from build123d import *

# Parameters (mm, degrees)
SKETCH2_R               = 34
BOSS_EXTRUDE1_DEPTH     = 5
CUT_EXTRUDE_THIN1_REACH = 50.343
CUT_EXTRUDE1_REACH      = 50.343
SKETCH7_R               = 1.5
CUT_EXTRUDE2_REACH      = 50.343
SKETCH8_R               = 3.5
SKETCH9_R               = 30
CUT_EXTRUDE3_DEPTH      = 2


with BuildPart() as part:
    # Sketch2 → Boss-Extrude1 (new body)
    with BuildSketch(Plane.XY):
        Circle(SKETCH2_R)
    extrude(amount=BOSS_EXTRUDE1_DEPTH)

    # Sketch3 → Cut-Extrude-Thin1 (cut, up to next)
    with BuildSketch(Plane.XY.offset(5), mode=Mode.PRIVATE) as cut_extrude_thin1_sk1:
        with BuildLine():
            ThreePointArc((0, 25.5), (18, 7.5), (0, -10.5))
            Line((0, -10.5), (0, -17.5))
            ThreePointArc((0, -17.5), (25, 7.5), (0, 32.5))
            Line((0, 32.5), (0, 25.5))
        make_face()
    cut_extrude_thin1_tool1 = extrude(cut_extrude_thin1_sk1.sketch, amount=-CUT_EXTRUDE_THIN1_REACH, mode=Mode.PRIVATE) & part.part
    # Sketch3 → Cut-Extrude-Thin1 (cut, up to next)
    with BuildSketch(Plane.XY.offset(5), mode=Mode.PRIVATE) as cut_extrude_thin1_sk2:
        with BuildLine():
            ThreePointArc((22.083647797, -12.75), (-2.504809472, -19.338457268), (-9.09326674, 5.25))
            Line((-9.09326674, 5.25), (-15.155444566, 8.75))
            ThreePointArc((-15.155444566, 8.75), (-6.004809472, -25.400635095), (28.145825623, -16.25))
            Line((28.145825623, -16.25), (22.083647797, -12.75))
        make_face()
    cut_extrude_thin1_tool2 = extrude(cut_extrude_thin1_sk2.sketch, amount=-CUT_EXTRUDE_THIN1_REACH, mode=Mode.PRIVATE) & part.part
    # Sketch3 → Cut-Extrude-Thin1 (cut, up to next)
    with BuildSketch(Plane.XY.offset(5), mode=Mode.PRIVATE) as cut_extrude_thin1_sk3:
        with BuildLine():
            ThreePointArc((-22.083647797, -12.75), (-15.495190528, 11.838457268), (9.09326674, 5.25))
            Line((9.09326674, 5.25), (15.155444566, 8.75))
            ThreePointArc((15.155444566, 8.75), (-18.995190528, 17.900635095), (-28.145825623, -16.25))
            Line((-28.145825623, -16.25), (-22.083647797, -12.75))
        make_face()
    cut_extrude_thin1_tool3 = extrude(cut_extrude_thin1_sk3.sketch, amount=-CUT_EXTRUDE_THIN1_REACH, mode=Mode.PRIVATE) & part.part
    add(cut_extrude_thin1_tool1.solids().sort_by_distance((0.559017, 29, 5))[0], mode=Mode.SUBTRACT)
    add(cut_extrude_thin1_tool2.solids().sort_by_distance((-2.804081, -19.85681, 5))[0], mode=Mode.SUBTRACT)
    add(cut_extrude_thin1_tool3.solids().sort_by_distance((-15.794462, 12.35681, 5))[0], mode=Mode.SUBTRACT)

    # Sketch7 → Cut-Extrude1 (cut, up to next)
    with BuildSketch(Plane(origin=(0, 0, 0), x_dir=(-1, 0, 0), z_dir=(0, 0, -1)), mode=Mode.PRIVATE) as cut_extrude1_sk1:
        with Locations((7, 0)):
            Circle(SKETCH7_R)
    cut_extrude1_tool1 = extrude(cut_extrude1_sk1.sketch, amount=-CUT_EXTRUDE1_REACH, mode=Mode.PRIVATE) & part.part
    # Sketch7 → Cut-Extrude1 (cut, up to next)
    with BuildSketch(Plane(origin=(0, 0, 0), x_dir=(-1, 0, 0), z_dir=(0, 0, -1)), mode=Mode.PRIVATE) as cut_extrude1_sk2:
        with Locations((0, -7)):
            Circle(SKETCH7_R)
    cut_extrude1_tool2 = extrude(cut_extrude1_sk2.sketch, amount=-CUT_EXTRUDE1_REACH, mode=Mode.PRIVATE) & part.part
    # Sketch7 → Cut-Extrude1 (cut, up to next)
    with BuildSketch(Plane(origin=(0, 0, 0), x_dir=(-1, 0, 0), z_dir=(0, 0, -1)), mode=Mode.PRIVATE) as cut_extrude1_sk3:
        with Locations((-7, 0)):
            Circle(SKETCH7_R)
    cut_extrude1_tool3 = extrude(cut_extrude1_sk3.sketch, amount=-CUT_EXTRUDE1_REACH, mode=Mode.PRIVATE) & part.part
    # Sketch7 → Cut-Extrude1 (cut, up to next)
    with BuildSketch(Plane(origin=(0, 0, 0), x_dir=(-1, 0, 0), z_dir=(0, 0, -1)), mode=Mode.PRIVATE) as cut_extrude1_sk4:
        with Locations((0, 7)):
            Circle(SKETCH7_R)
    cut_extrude1_tool4 = extrude(cut_extrude1_sk4.sketch, amount=-CUT_EXTRUDE1_REACH, mode=Mode.PRIVATE) & part.part
    add(cut_extrude1_tool1.solids().sort_by_distance((-7, 0, 0))[0], mode=Mode.SUBTRACT)
    add(cut_extrude1_tool2.solids().sort_by_distance((0, -7, 0))[0], mode=Mode.SUBTRACT)
    add(cut_extrude1_tool3.solids().sort_by_distance((7, 0, 0))[0], mode=Mode.SUBTRACT)
    add(cut_extrude1_tool4.solids().sort_by_distance((0, 7, 0))[0], mode=Mode.SUBTRACT)

    # Sketch8 → Cut-Extrude2 (cut, up to next)
    with BuildSketch(Plane(origin=(0, 0, 0), x_dir=(-1, 0, 0), z_dir=(0, 0, -1)), mode=Mode.PRIVATE) as cut_extrude2_sk1:
        with Locations((0, 29)):
            Circle(SKETCH8_R)
    cut_extrude2_tool1 = extrude(cut_extrude2_sk1.sketch, amount=-CUT_EXTRUDE2_REACH, mode=Mode.PRIVATE) & part.part
    # Sketch8 → Cut-Extrude2 (cut, up to next)
    with BuildSketch(Plane(origin=(0, 0, 0), x_dir=(-1, 0, 0), z_dir=(0, 0, -1)), mode=Mode.PRIVATE) as cut_extrude2_sk2:
        with Locations((-12.124355653, 7)):
            Circle(SKETCH8_R)
    cut_extrude2_tool2 = extrude(cut_extrude2_sk2.sketch, amount=-CUT_EXTRUDE2_REACH, mode=Mode.PRIVATE) & part.part
    # Sketch8 → Cut-Extrude2 (cut, up to next)
    with BuildSketch(Plane(origin=(0, 0, 0), x_dir=(-1, 0, 0), z_dir=(0, 0, -1)), mode=Mode.PRIVATE) as cut_extrude2_sk3:
        with Locations((12.124355653, 7)):
            Circle(SKETCH8_R)
    cut_extrude2_tool3 = extrude(cut_extrude2_sk3.sketch, amount=-CUT_EXTRUDE2_REACH, mode=Mode.PRIVATE) & part.part
    # Sketch8 → Cut-Extrude2 (cut, up to next)
    with BuildSketch(Plane(origin=(0, 0, 0), x_dir=(-1, 0, 0), z_dir=(0, 0, -1)), mode=Mode.PRIVATE) as cut_extrude2_sk4:
        with Locations((25.11473671, -14.5)):
            Circle(SKETCH8_R)
    cut_extrude2_tool4 = extrude(cut_extrude2_sk4.sketch, amount=-CUT_EXTRUDE2_REACH, mode=Mode.PRIVATE) & part.part
    # Sketch8 → Cut-Extrude2 (cut, up to next)
    with BuildSketch(Plane(origin=(0, 0, 0), x_dir=(-1, 0, 0), z_dir=(0, 0, -1)), mode=Mode.PRIVATE) as cut_extrude2_sk5:
        with Locations((-25.11473671, -14.5)):
            Circle(SKETCH8_R)
    cut_extrude2_tool5 = extrude(cut_extrude2_sk5.sketch, amount=-CUT_EXTRUDE2_REACH, mode=Mode.PRIVATE) & part.part
    # Sketch8 → Cut-Extrude2 (cut, up to next)
    with BuildSketch(Plane(origin=(0, 0, 0), x_dir=(-1, 0, 0), z_dir=(0, 0, -1)), mode=Mode.PRIVATE) as cut_extrude2_sk6:
        with Locations((0, -14)):
            Circle(SKETCH8_R)
    cut_extrude2_tool6 = extrude(cut_extrude2_sk6.sketch, amount=-CUT_EXTRUDE2_REACH, mode=Mode.PRIVATE) & part.part
    add(cut_extrude2_tool1.solids().sort_by_distance((0, 29, 0))[0], mode=Mode.SUBTRACT)
    add(cut_extrude2_tool2.solids().sort_by_distance((12.124356, 7, 0))[0], mode=Mode.SUBTRACT)
    add(cut_extrude2_tool3.solids().sort_by_distance((-12.124356, 7, 0))[0], mode=Mode.SUBTRACT)
    add(cut_extrude2_tool4.solids().sort_by_distance((-25.114737, -14.5, 0))[0], mode=Mode.SUBTRACT)
    add(cut_extrude2_tool5.solids().sort_by_distance((25.114737, -14.5, 0))[0], mode=Mode.SUBTRACT)
    add(cut_extrude2_tool6.solids().sort_by_distance((0, -14, 0))[0], mode=Mode.SUBTRACT)

    # Sketch9 → Cut-Extrude3 (cut)
    with BuildSketch(Plane(origin=(0, 0, 0), x_dir=(-1, 0, 0), z_dir=(0, 0, -1))):
        Circle(SKETCH9_R)
    extrude(amount=-CUT_EXTRUDE3_DEPTH, mode=Mode.SUBTRACT)


solid = part.part
CAD build for the part. Positions are in the model's coordinates, mm. A direction names the side the tool comes from. Round coordinates to 2 decimals unless told otherwise and drop trailing zeros. Loops run counter-clockwise (first coordinate to the right, second up) from the corner with the lowest first, then second, coordinate; pieces in that order, holes last.
(1) Wall check: line 1 along Y through (x, z) = (16.5, 2.3); line 2 along X through (y, z) = (8, 3.4) (3 decimals); line 3 along Y through (x, z) = (6, 2.6). Give the ranges that are in metal, low to high.
(2) Cut at B-B (x = -17). Give the cut face in (y, z).
(3) Two-plate mould, pull along Y, no slides. Class faces 1 (the cylindrical face through (18.28, 28.67, 2.46)), 2 (the cylindrical face through (17.996, 7.896, 3.521)), 3 (the flat face through (2.4, -30.1, 0)): +Y half, -Y half, draft (parallel to the pull), parting line (faces both ways), or undercut.
(4) Cut at C-C (y = -14). Give the cut face in (x, z), plus the area to 3 significant figures.
(5) Which spindle directions (+Z, -Z, +X, -X, +Y, -Y) get a long thin tool onto all of the face, cutting with end or side? Do faces 4 (the cylindrical face through (-3.5, -14.1, 3.5)), 5 (the cylindrical face through (-20.251, 22.134, 0.986)). Say none if no direction does.
(6) Cut at A-A (y = -3.5). Give the cut face in (x, z), plus the area to 3 significant figures.
(7) Drop flat-ended pins along their axis: pin 1 (5 mm diameter, centred on x = -7, y = 0, fed in from -Z); pin 2 (2 mm diameter, centred on x = -26.5, z = 3.5, fed in from -Y); pin 3 (5 mm diameter, centred on x = 0, y = 7, fed in from +Z); pin 4 (3 mm diameter, centred on x = 3, y = -15, fed in from -Z). Give the stop position or say it passes through.
Findings below:
1. line 1: y = -29.73 to -26.66, -18.71 to -11.28, 0.31 to 14.69, 26.28 to 29.73
1. line 2: x = -33.045 to -28.562, -20.131 to -15.571, -8.77 to -1.118, 1.118 to 7.141, 15.478 to 17.993, 24.995 to 33.045
1. line 3: y = -33.47 to -28.75, -21.74 to -16.77, -9.47 to -1.12, 1.12 to 9.21, 17.9 to 24.47, 31.77 to 33.47
2. outline: (-29.44, 0) - (-24.72, 0) - (-24.72, 2) - (-12.29, 2) - (-12.29, 5) - (-29.44, 5) - close; (4.79, 2) - (10.87, 2) - (10.87, 5) - (4.79, 5) - close; (18.94, 2) - (24.72, 2) - (24.72, 0) - (29.44, 0) - (29.44, 5) - (18.94, 5) - close
3. face 1: parting line
3. face 2: undercut
3. face 3: draft
4. outline: (-30.98, 0) - (-29.3, 0) - (-29.3, 5) - (-30.98, 5) - close; (-21.65, 2) - (-16.31, 2) - (-16.31, 5) - (-21.65, 5) - close; (-8.3, 2) - (-3.5, 2) - (-3.5, 5) - (-8.3, 5) - close; (12.76, 2) - (21.29, 2) - (21.29, 5) - (12.76, 5) - close; (28.58, 0) - (30.98, 0) - (30.98, 5) - (28.58, 5) - close
4. area: 76.5 mm2
5. face 4: +Z, -Z
5. face 5: -Z
6. outline: (-33.82, 0) - (-31.49, 0) - (-31.49, 5) - (-33.82, 5) - close; (-24.49, 2) - (-18.5, 2) - (-18.5, 5) - (-24.49, 5) - close; (-11.5, 2) - (14.25, 2) - (14.25, 5) - (-11.5, 5) - close; (22.45, 2) - (29.8, 2) - (29.8, 0) - (33.82, 0) - (33.82, 5) - (22.45, 5) - close
6. area: 149 mm2
7. pin 1: stops at z = 2
7. pin 2: stops at y = -22.49
7. pin 3: stops at z = 5
7. pin 4: passes through
